The model under review builds one solid part; all positions refer to its coordinate system, in mm. A direction names the side the tool comes from. Round coordinates to 2 decimals unless told otherwise and drop trailing zeros. Write each loop counter-clockwise with the first axis right and the second up, starting at its lowest first coordinate (ties: lowest second). Pieces come first, ordered by that corner, then holes. Notation, with made-up numbers: (52.25, -38.75) - (82.25, -38.75) arc R13 ccw to (82.25, -21.75) - close; hole circle Ø7 at (10.5, -31). An arc over 180 degrees is marked (long way). Use one line per item in the form item = value.
from build123d import *

# Parameters (mm, degrees)
SKETCH1_R           = 5
BOSS_EXTRUDE1_DEPTH = 62
SKETCH3_W           = 15.25
SKETCH3_H           = 15.25
BOSS_EXTRUDE2_DEPTH = 30
SKETCH5_R           = 3
CUT_EXTRUDE1_DEPTH  = 10
SKETCH4_R           = 2.75
BOSS_EXTRUDE3_DEPTH = 34


with BuildPart() as part:
    # Sketch1 → Boss-Extrude1 (new body)
    with BuildSketch(Plane(origin=(0, 0, 0), x_dir=(1, 0, 0), z_dir=(0, 1, 0))):
        with Locations(Location((0, 0, 0), (0, 0, 270))):
            Circle(SKETCH1_R)
    extrude(amount=BOSS_EXTRUDE1_DEPTH)

    # Sketch3 → Boss-Extrude2 (add)
    with BuildSketch(Plane(origin=(0, 62, 0), x_dir=(1, 0, 0), z_dir=(0, 1, 0))):
        Rectangle(SKETCH3_W, SKETCH3_H)
    extrude(amount=BOSS_EXTRUDE2_DEPTH)

    # Sketch5 → Cut-Extrude1 (cut)
    with BuildSketch(Plane.XZ):
        with Locations(Location((0, 0, 0), (0, 0, 270))):
            Circle(SKETCH5_R)
    extrude(amount=-CUT_EXTRUDE1_DEPTH, mode=Mode.SUBTRACT)

    # Sketch4 → Boss-Extrude3 (add)
    with BuildSketch(Plane(origin=(0, 92, 0), x_dir=(1, 0, 0), z_dir=(0, 1, 0))):
        with Locations(Location((0, 0, 0), (0, 0, 270))):
            Circle(SKETCH4_R)
    extrude(amount=BOSS_EXTRUDE3_DEPTH)


solid = part.part
(1) Add section A-A on z = 0. Write out the cut boundary in (x, y) (3 decimals), then the cut area to 3 significant figures.
Geometry results:
outline = (-7.625, 62) - (-5, 62) - (-5, 0) - (-3, 0) - (-3, 10) - (3, 10) - (3, 0) - (5, 0) - (5, 62) - (7.625, 62) - (7.625, 92) - (2.75, 92) - (2.75, 126) - (-2.75, 126) - (-2.75, 92) - (-7.625, 92) - close
area = 1,200 mm2
(2) To check wall thickness, follow L1, parallel to X at y = 4.5, z = 0; L2, parallel to Y at x = -5.5, z = 5.5; L3, parallel to Y at x = 1.5, z = 0.5. State the ranges of each line that lie inside material, in increasing order.
Geometry results:
L1 = -5 to -3, 3 to 5
L2 = 62 to 92
L3 = 10 to 126
(3) Add section C-C on z = -6.5. Write out the cut boundary in (x, y) (3 decimals).
Geometry results:
outline = (-7.625, 62) - (7.625, 62) - (7.625, 92) - (-7.625, 92) - close
(4) The part is to be moulded in two halves that separate along Z. For faces 4 (the flat face through (0, 10, 0)), 5 (the flat face through (0, 126, 0)), 6 (the flat face through (0, 77, 7.625)), 7 (the cylindrical face through (0.9, 4.93, -2.86)), say which applies: +Z half, -Z half, draft (parallel to the pull), parting line (faces both ways), or undercut.
Geometry results:
face_4 = undercut
face_5 = draft
face_6 = +Z half
face_7 = undercut
(5) Machinability: for faces 1 (the flat face through (-3.3, 0, -0.1)), 2 (the cylindrical face through (-4.88, 30.57, -1.08)), 3 (the cylindrical face through (-2.685, 108.762, -0.596)), which of the approach directions +Z, -Z, +X, -X, +Y, -Y give a long, thin tool a straight path to every point of the face, cutting with its end or side? Answer none if there is none.
Geometry results:
face_1 = +Z, -Z, +X, -X, -Y
face_2 = -Y
face_3 = +Y
(6) Insertion check: P1, Ø1, axis at y = 26, z = -3.5, coming from the -X side; P2, Ø4, axis at y = 47, z = -4, coming from the +X side; P3, Ø5, axis at y = 112, z = 1, coming from the -X side. Each pin has a flat end and moves straight along its axis. Give the tip position at first contact, or say it passes through.
Geometry results:
P1 = -4
P2 = 4.58
P3 = -2.75
(7) Add section B-B on y = 97.5. Write out the cut boundary in (x, z).
Geometry results:
outline = circle Ø5.5 at (0, 0)
